from build123d import *

# Parameters (mm, degrees)
F0_W      = 93.98
F0_H      = 207.01
F0_W_2    = 81.28
F0_H_2    = 87.122
F0_H_3    = 104.648
F1_DEPTH  = 63.5
F2_W      = 17.78
F2_H      = 50.8
F3_DEPTH  = 6.35
F4_W      = 25.4
F4_H      = 20.32
F5_DEPTH  = 38.1
F6_W      = 25.4
F6_H      = 25.4
F7_DEPTH  = 2.54
F9_DEPTH  = 25.4
F10_W     = 81.28
F10_H     = 2.54
F11_DEPTH = 63.5
F12_W     = 38.1
F12_H     = 50.8
F13_DEPTH = 25.4
F14_W     = 17.78
F14_H     = 20.32
F15_DEPTH = 38.1


with BuildPart() as f1:
    # F0 (on Front) → F1 (new body)
    with BuildSketch(Plane.XZ):
        with Locations((40.64, 97.155)):
            Rectangle(F0_W, F0_H)
        with Locations((40.64, 43.561)):
            Rectangle(F0_W_2, F0_H_2, mode=Mode.SUBTRACT)
        with Locations((40.64, 141.986)):
            Rectangle(F0_W_2, F0_H_3, mode=Mode.SUBTRACT)
    extrude(amount=F1_DEPTH)

    # F2 (on face) → F3 (cut, through all)
    with BuildSketch(Plane(origin=(0, 0, -6.35), x_dir=(1, 0, 0), z_dir=(0, 0, -1))):
        with Locations((15.24, 38.1)):
            Rectangle(F2_W, F2_H)
    extrude(amount=-F3_DEPTH, mode=Mode.SUBTRACT)

    # F4 (on face) → F5 (join)
    with BuildSketch(Plane.XZ.offset(63.5)):
        with Locations((12.7, 99.822)):
            Rectangle(F4_W, F4_H)
    extrude(amount=-F5_DEPTH)

    # F6 (on face) → F7 (cut, through all)
    with BuildSketch(Plane.XY.offset(89.662)):
        with Locations((12.7, -12.7)):
            Rectangle(F6_W, F6_H)
    extrude(amount=-F7_DEPTH, mode=Mode.SUBTRACT)

    # F8 (on face) → F9 (join, through all)
    with BuildSketch(Plane.YZ):
        Polygon((-33.02, 79.502), (-33.02, 87.122), (-63.5, 87.122), (-63.5, 56.642), (-55.88, 56.642), (-55.88, 64.262), (-48.26, 64.262), (-48.26, 71.882), (-40.64, 71.882), (-40.64, 79.502), align=None)
    extrude(amount=F9_DEPTH)

    # F10 (on face) → F11 (join, through all)
    with BuildSketch(Plane.XZ.offset(63.5)):
        with Locations((40.64, 111.252)):
            Rectangle(F10_W, F10_H)
    extrude(amount=-F11_DEPTH)

    # F12 (on face) → F13 (cut, through all)
    with BuildSketch(Plane(origin=(0, 0, 87.122), x_dir=(1, 0, 0), z_dir=(0, 0, -1))):
        with Locations((62.23, 38.1)):
            Rectangle(F12_W, F12_H)
    extrude(amount=-F13_DEPTH, mode=Mode.SUBTRACT)

    # F14 (on face) → F15 (join, through all)
    with BuildSketch(Plane.XZ.offset(63.5)):
        with Locations((34.29, 99.822)):
            Rectangle(F14_W, F14_H)
    extrude(amount=-F15_DEPTH)


solid = f1.part
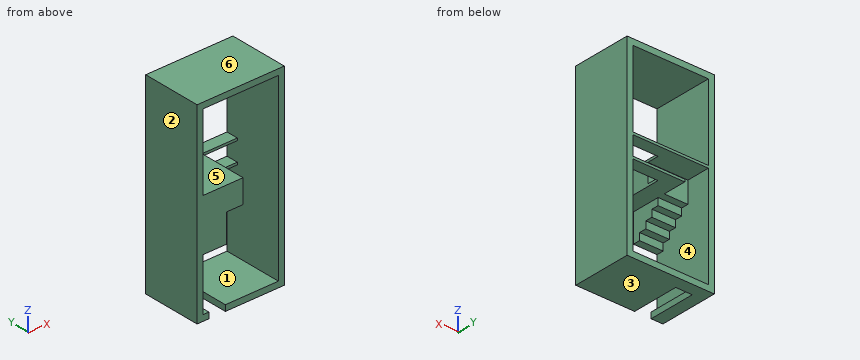
Geometry check sheet. Reference: the model listing, model coordinates, mm. Face numbers are marked on the shaded views. A direction names the side the tool comes from. Round coordinates to 2 decimals unless told otherwise and drop trailing zeros. Write each loop counter-clockwise with the first axis right and the second up, starting at its lowest first coordinate (ties: lowest second). Pieces come first, ordered by that corner, then holes. Notation, with made-up numbers: (-15.5, 25) -> (39.5, 25) arc R6 cw to (39.5, 30) -> close; hole circle Ø10 at (24, -24). An arc over 180 degrees is marked (long way). One line per item, written item: value. Start each with the question number.
(1) Scan lines: line 1 (Z direction, x = 37.5, y = -34); line 2 (Z direction, x = 71, y = -9); line 3 (Z direction, x = 4.5, y = -22). Record each from-to range of solid material in increasing order. Write a range as [from, to].
(2) Access from +Z, -Z, +X, -X, +Y, -Y to the whole of each face (thin tool, end or side, straight path). Record for the marked faces 4, 5 and 6.
(3) Draft check along X on the marked faces 1, 2 and 3. Enter one of: +X half, -X half, draft (parallel to the pull), parting line (faces both ways), or undercut.
(4) Cross-section at B-B, the plane x = 58. Record the cut outline in (y, z), and give its area (3 significant figures).
(5) Cross-section at D-D, the plane z = 105. Record the cut outline in (x, y).
(6) Cross-section at A-A, the plane y = -20.5. Record the cut outline in (x, z), and give its area (3 significant figures).
(7) Cross-section at C-C, the plane y = -5.5. Record the cut outline in (x, z).
(8) Go/stop test with flat-tipped pins: pin 1 Ø7 at (x, z) = (19, -2) entering from -Y; pin 2 Ø8.5 at (x, z) = (18, 75) entering from +Y; pin 3 Ø4 at (x, y) = (15, -35) entering from -Z. Record where each tip stops, or that it passes through.
Answer:
1. line 1: [-6.35, 0], [87.12, 112.52], [194.31, 200.66]
1. line 2: [-6.35, 0], [87.12, 89.66], [109.98, 112.52], [194.31, 200.66]
1. line 3: [-6.35, 0], [109.98, 112.52], [194.31, 200.66]
2. face 4: +Y
2. face 5: +Y, -Y
2. face 6: +Z, +X, -X, +Y, -Y
3. face 1: undercut
3. face 2: -X half
3. face 3: draft
4. outline: (-63.5, -6.35) -> (0, -6.35) -> (0, 0) -> (-63.5, 0) -> close; (-63.5, 194.31) -> (0, 194.31) -> (0, 200.66) -> (-63.5, 200.66) -> close; (-12.7, 87.12) -> (0, 87.12) -> (0, 89.66) -> (-12.7, 89.66) -> close; (-12.7, 109.98) -> (0, 109.98) -> (0, 112.52) -> (-12.7, 112.52) -> close
4. area: 871 mm²
5. outline: (-6.35, -63.5) -> (43.18, -63.5) -> (43.18, -25.4) -> (0, -25.4) -> (0, 0) -> (-6.35, 0) -> close; (81.28, -63.5) -> (87.63, -63.5) -> (87.63, 0) -> (81.28, 0) -> close
6. outline: (-6.35, -6.35) -> (6.35, -6.35) -> (6.35, 0) -> (0, 0) -> (0, 109.98) -> (43.18, 109.98) -> (43.18, 112.52) -> (0, 112.52) -> (0, 194.31) -> (81.28, 194.31) -> (81.28, 0) -> (24.13, 0) -> (24.13, -6.35) -> (87.63, -6.35) -> (87.63, 200.66) -> (-6.35, 200.66) -> close; (25.4, 87.12) -> (43.18, 87.12) -> (43.18, 89.66) -> (25.4, 89.66) -> close
6. area: 3,700 mm²
7. outline: (-6.35, -6.35) -> (87.63, -6.35) -> (87.63, 200.66) -> (-6.35, 200.66) -> close; hole (0, 0) -> (81.28, 0) -> (81.28, 87.12) -> (25.4, 87.12) -> (25.4, 89.66) -> (81.28, 89.66) -> (81.28, 109.98) -> (0, 109.98) -> close; hole (0, 112.52) -> (81.28, 112.52) -> (81.28, 194.31) -> (0, 194.31) -> close
8. pin 1: y = -12.7
8. pin 2: y = -40.64
8. pin 3: z = 79.5
